The listing builds one solid part. Answer for the finished solid, in the listing's coordinates (mm). Face numbers are marked on the shaded views. A direction names the side the tool comes from. Give positions to 0.01 mm unless a question says otherwise; leave off trailing zeros. Write each loop counter-clockwise with the first axis right and the second up, starting at its lowest first coordinate (ties: lowest second). Pieces come first, ordered by that corner, then holes. Notation, with made-up numbers: (-21.5, 24.25) -> (-15.5, 24.25) arc R27 cw to (-15.5, 52.25) -> close; hole circle Ø2 at (69.25, 25). An arc over 180 degrees is marked (long way). Put each result on its own line as item: value. Start each with the question number.
1) Flat-ended cylindrical pins translate along their axes: pin 1 Ø3 at (x, z) = (-7, -19.5) entering from +Y; pin 2 Ø3 at (y, z) = (-7.31, -30) entering from +X; pin 3 Ø2.5 at (x, y) = (-3.5, -35) entering from -Z; pin 4 Ø5 at (y, z) = (5.5, -6.5) entering from +X. Find the tip coordinate at first contact, or state that the pin passes through.
2) Find the intervals of material crossed by line 1 along Z through (x, y) = (125, -36); line 2 along X through (y, z) = (40, -11); line 3 along X through (y, z) = (-34.4, -22), in increasing order. Write a range as from..to.
3) A cutting plane is placed at B-B (x = 125). Write down the section's boundary in (y, z), then the cut area to 3 significant figures.
4) A cutting plane is placed at C-C (y = 21.5). Write down the section's boundary in (x, z), then the cut area to 3 significant figures.
5) For the marked faces 1, 2 and 3, determine the directions among +Z, -Z, +X, -X, +Y, -Y from which every point of the face is accessible in a straight line to the end or side of a thin tool.
6) For a pull along Y with two mould halves and no side action, classify the marked faces 4, 5 and 6 as released by +Y, released by -Y, zero draft, split by the parting line, or undercut.
7) A cutting plane is placed at D-D (x = -5). Write down the section's boundary in (y, z), then the cut area to 3 significant figures.
8) A cutting plane is placed at A-A (y = -25.5). Write down the section's boundary in (x, z), then the cut area to 3 significant figures.
from build123d import *

# Parameters (mm, degrees)
ESQUISSE4_R             = 2
ESQUISSE4_R_2           = 5
BOSS_EXTRU_1_DEPTH      = 120
ESQUISSE19_W            = 107
ESQUISSE19_H            = 83.7
ENL_V_MAT_EXTRU_1_DEPTH = 120
ESQUISSE20_R            = 16.25
ESQUISSE20_R_2          = 14
BOSS_EXTRU_2_DEPTH      = 21.5
ESQUISSE28_W            = 19
ESQUISSE28_H            = 5
BOSS_EXTRU_6_DEPTH      = 10
ESQUISSE29_R            = 1.75
ENL_V_MAT_EXTRU_6_DEPTH = 10
ESQUISSE33_W            = 19
ESQUISSE33_H            = 5
BOSS_EXTRU_7_DEPTH      = 10
ESQUISSE34_R            = 1.975077454
ESQUISSE34_R_2          = 2.125479737
ENL_V_MAT_EXTRU_7_DEPTH = 159.52662237


with BuildPart() as part:
    # Esquisse4 → Boss.-Extru.1 (new body)
    with BuildSketch(Plane(origin=(0, 0, 0), x_dir=(0, 0, -1), z_dir=(1, 0, 0))):
        Polygon((30, -37.604112468), (35, -37.604112468), (35, 51.095887532), (0, 51.095887532), (0, -37.604112468), align=None)
        with Locations((30, -7.314112468)):
            Circle(ESQUISSE4_R, mode=Mode.SUBTRACT)
        with Locations((18.58577647, 18.253748241)):
            Circle(ESQUISSE4_R_2, mode=Mode.SUBTRACT)
    extrude(amount=BOSS_EXTRU_1_DEPTH)

    # Esquisse19 → Enlèv. mat.-Extru.1 (cut)
    with BuildSketch(Plane(origin=(0, 0, -35), x_dir=(-1, 0, 0), z_dir=(0, 0, -1))):
        with Locations((-60, 4.245887532)):
            Rectangle(ESQUISSE19_W, ESQUISSE19_H)
    extrude(amount=-ENL_V_MAT_EXTRU_1_DEPTH, mode=Mode.SUBTRACT)

    # Esquisse20 → Boss.-Extru.2 (add)
    with BuildSketch(Plane(origin=(120, 0, 0), x_dir=(0, 0, -1), z_dir=(1, 0, 0))):
        with Locations((18.58577647, 18.253748241)):
            Circle(ESQUISSE20_R)
        with Locations((18.58577647, 18.253748241)):
            Circle(ESQUISSE20_R_2, mode=Mode.SUBTRACT)
    extrude(amount=-BOSS_EXTRU_2_DEPTH)

    # Esquisse28 → Boss.-Extru.6 (add)
    with BuildSketch(Plane(origin=(120, 0, 0), x_dir=(0, 0, -1), z_dir=(1, 0, 0))):
        with Locations((17.5, -35.104112468)):
            Rectangle(ESQUISSE28_W, ESQUISSE28_H)
    extrude(amount=BOSS_EXTRU_6_DEPTH)

    # Esquisse29 → Enlèv. mat.-Extru.6 (cut)
    with BuildSketch(Plane(origin=(0, -32.604112468, 0), x_dir=(1, 0, 0), z_dir=(0, 1, 0))):
        with Locations(Location((125, 22, 0), (0, 0, 270))):
            Circle(ESQUISSE29_R)
        with Locations(Location((125, 13, 0), (0, 0, 270))):
            Circle(ESQUISSE29_R)
    extrude(amount=-ENL_V_MAT_EXTRU_6_DEPTH, mode=Mode.SUBTRACT)

    # Esquisse33 → Boss.-Extru.7 (add)
    with BuildSketch(Plane.ZY):
        with Locations((-17.5, -35.104112468)):
            Rectangle(ESQUISSE33_W, ESQUISSE33_H)
    extrude(amount=BOSS_EXTRU_7_DEPTH)

    # Esquisse34 → Enlèv. mat.-Extru.7 (cut, through all)
    with BuildSketch(Plane(origin=(0, -32.604112468, 0), x_dir=(1, 0, 0), z_dir=(0, 1, 0))):
        with Locations(Location((-5, 22, 0), (0, 0, 270))):
            Circle(ESQUISSE34_R)
        with Locations(Location((-5, 13, 0), (0, 0, 270))):
            Circle(ESQUISSE34_R_2)
    extrude(amount=-ENL_V_MAT_EXTRU_7_DEPTH, mode=Mode.SUBTRACT)


solid = part.part
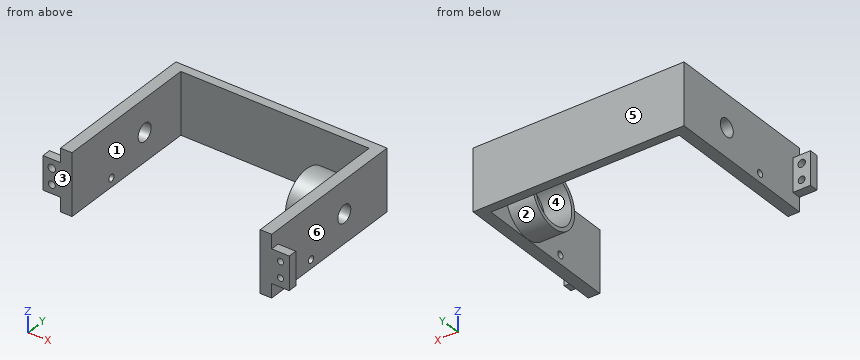
Reply:
1. pin 1: stops at y = -32.6
1. pin 2: passes through
1. pin 3: stops at z = -27
1. pin 4: stops at x = 120
2. line 1: z = -27..-23.75, -20.25..-14.75, -11.25..-8
2. line 2: x = 0..6.5, 113.5..120
2. line 3: x = -10..-6.98, -3.02..6.5, 113.5..123.25, 126.75..130
3. outline: (-37.6, -27) -> (-32.6, -27) -> (-32.6, -23.75) -> (-37.6, -23.75) -> close; (-37.6, -20.25) -> (-32.6, -20.25) -> (-32.6, -14.75) -> (-37.6, -14.75) -> close; (-37.6, -11.25) -> (-32.6, -11.25) -> (-32.6, -8) -> (-37.6, -8) -> close
3. area: 60.0 mm2
4. outline: (0, -35) -> (6.5, -35) -> (6.5, -22.39) -> (0, -22.39) -> close; (0, -14.78) -> (6.5, -14.78) -> (6.5, 0) -> (0, 0) -> close; (98.5, -34.51) -> (113.5, -34.51) -> (113.5, -35) -> (120, -35) -> (120, -22.39) -> (113.5, -22.39) -> (113.5, -32.2) -> (98.5, -32.2) -> close; (98.5, -4.97) -> (113.5, -4.97) -> (113.5, -14.78) -> (120, -14.78) -> (120, 0) -> (113.5, 0) -> (113.5, -2.66) -> (98.5, -2.66) -> close
4. area: 425 mm2
5. face 1: +Z, -Z, -Y
5. face 2: none
5. face 3: +Z, -Z, +X, -X, -Y
6. face 4: undercut
6. face 5: released by +Y
6. face 6: zero draft
7. outline: (-37.6, -27) -> (-32.6, -27) -> (-32.6, -23.98) -> (-37.6, -23.98) -> close; (-37.6, -20.02) -> (-32.6, -20.02) -> (-32.6, -15.13) -> (-37.6, -15.13) -> close; (-37.6, -10.87) -> (-32.6, -10.87) -> (-32.6, -8) -> (-37.6, -8) -> close
7. area: 54.0 mm2
8. outline: (0, -35) -> (6.5, -35) -> (6.5, 0) -> (0, 0) -> close; (113.5, -35) -> (120, -35) -> (120, 0) -> (113.5, 0) -> close
8. area: 455 mm2
